```python
from build123d import *

# Parameters (mm, degrees)
SKETCH1_W                                 = 241.3
SKETCH1_H                                 = 177.8
BASE_FLANGE1_DEPTH                        = 3.175
EDGE_FLANGE1_DEPTH                        = 177.8
EDGE_FLANGE1_BEND_DEPTH                   = 177.8
SKETCH13_W                                = 136.525
SKETCH13_H                                = 12.7
BOSS_EXTRUDE1_DEPTH                       = 3.175
SKETCH39_W                                = 136.525
SKETCH39_H                                = 12.7
BOSS_EXTRUDE2_DEPTH                       = 3.175
HOLE_FOR_1_4_SELF_CLINCHING_NUTS_S_SS_C_D = 8.7376
FILLET2_R                                 = 4.7625


# Sheet-metal steps are written as plain solids
with BuildPart() as part:
    # Sketch1 → Base-Flange1 (new body)
    with BuildSketch(Plane(origin=(0, 0, 0), x_dir=(1, 0, 0), z_dir=(0, 1, 0))):
        Rectangle(SKETCH1_W, SKETCH1_H)
    extrude(amount=-BASE_FLANGE1_DEPTH)

    # Edge-Flange1 section (across the edge) → Edge-Flange1 (add)
    with BuildSketch(Plane(origin=(123.825, -3.175, -88.9), x_dir=(-1, 0, 0), z_dir=(0, 0, 1))):
        with BuildLine():
            Line((-3.175, 3.175), (-3.175, 22.225))
            Line((-3.175, 22.225), (0, 22.225))
            Line((0, 22.225), (0, 3.175))
            ThreePointArc((0, 3.175), (0.92993597, 0.92993597), (3.175, 0))
            Line((3.175, 0), (3.175, -3.175))
            ThreePointArc((3.175, -3.175), (-1.315128061, -1.315128061), (-3.175, 3.175))
        make_face()
    extrude(amount=EDGE_FLANGE1_DEPTH)

    # Edge-Flange1 section 2 (across the edge) → Edge-Flange1 bend (add)
    with BuildSketch(Plane(origin=(-123.825, -3.175, 88.9), x_dir=(1, 0, 0), z_dir=(0, 0, -1))):
        with BuildLine():
            Line((-3.175, 3.175), (-3.175, 22.225))
            Line((-3.175, 22.225), (0, 22.225))
            Line((0, 22.225), (0, 3.175))
            ThreePointArc((0, 3.175), (0.92993597, 0.92993597), (3.175, 0))
            Line((3.175, 0), (3.175, -3.175))
            ThreePointArc((3.175, -3.175), (-1.315128061, -1.315128061), (-3.175, 3.175))
        make_face()
    extrude(amount=EDGE_FLANGE1_BEND_DEPTH)

    # Sketch13 → Boss-Extrude1 (add)
    with BuildSketch(Plane(origin=(127, 0, 0), x_dir=(0, 0, -1), z_dir=(1, 0, 0))):
        with Locations((0, -31.75)):
            Rectangle(SKETCH13_W, SKETCH13_H)
    extrude(amount=-BOSS_EXTRUDE1_DEPTH)

    # Sketch39 → Boss-Extrude2 (add)
    with BuildSketch(Plane.ZY.offset(127)):
        with Locations((0, -31.75)):
            Rectangle(SKETCH39_W, SKETCH39_H)
    extrude(amount=-BOSS_EXTRUDE2_DEPTH)

    # Hole for 1/4 Self-clinching Nuts (S,SS,CLS,CLSS)1 (through all)
    with Locations(Plane(origin=(127, 0, 0), x_dir=(0, 0, -1), z_dir=(1, 0, 0))):
        with Locations((-76.2, -15.875), (76.2, -15.875), (58.7375, -28.575), (-49.2125, -28.575)):
            Hole(HOLE_FOR_1_4_SELF_CLINCHING_NUTS_S_SS_C_D / 2)

    # Fillet2
    fillet2_edges = [part.edges().sort_by_distance(p)[0] for p in [
        (125.4125, -25.4, -88.9),
        (125.4125, -25.4, 88.9),
        (-125.4125, -25.4, 88.9),
        (-125.4125, -25.4, -88.9),
        (125.4125, -38.1, -68.2625),
        (125.4125, -25.4, -68.2625),
        (125.4125, -25.4, 68.2625),
        (125.4125, -38.1, 68.2625),
        (-125.4125, -25.4, -68.2625),
        (-125.4125, -38.1, -68.2625),
        (-125.4125, -38.1, 68.2625),
        (-125.4125, -25.4, 68.2625),
    ]]
    fillet(fillet2_edges, radius=FILLET2_R)


solid = part.part
```
Model file for the job. Use its own axes, mm. A direction names the side the tool comes from. Give positions to 0.01 mm unless a question says otherwise; leave off trailing zeros. Order: outer loops, then holes, each group sorted by start corner. A loop starts at its lowest first (then second) coordinate and runs counter-clockwise, first axis right, second up.
1) Saw through at C-C, the plane x = 51.5. Write the cut outline in (y, z) (3 decimals), then the cut area to 3 significant figures.
2) Saw through at A-A, the plane z = 76.2. Write the cut outline in (x, y) (3 decimals), then the cut area to 3 significant figures.
3) Pin check, flat tips, straight feed: pin 1 (2.5 mm diameter, centred on x = -124.5, y = -32, fed in from -Z); pin 2 (5 mm diameter, centred on y = -15.875, z = -76.2, fed in from +X); pin 3 (1.6 mm diameter, centred on x = -126, z = 78.5, fed in from -Y); pin 4 (3.5 mm diameter, centred on x = -125, y = -31.5, fed in from +Z). Stop position of each tip, or through.
4) Mould opens along Z. For faces 1 (the cylindrical face through (-125.435, -24.243, -59.306)), 2 (the cylindrical face through (125.39, -36.74, 66.83)), 3 (the cylindrical face through (125.09, -1.81, -1.24)), 4 (the flat face through (1, -2, -88.9)) say: +Z half, -Z half, draft (parallel to the pull), parting line (faces both ways), or undercut.
5) Saw through at B-B, the plane z = -15. Write the cut outline in (x, y) (3 decimals), then the cut area to 3 significant figures.
6) 3-axis set-ups, long thin cutter, end or side, ignore diameter. For faces 5 (the cylindrical face through (125.39, -18.53, -79.67)), 6 (the flat face through (-2, -3.175, -1)): which of +Z, -Z, +X, -X, +Y, -Y reach the whole face in a straight line?
7) Wall check: probe 1 along X at (y, z) = (-28, -30) (3 decimals); probe 2 along Y at (x, z) = (-89, 5) (3 decimals); probe 3 along X at (y, z) = (-4.5, 11). Give the ranges that are in metal, low to high.
Computed:
1. outline: (-3.175, -88.9) - (0, -88.9) - (0, 88.9) - (-3.175, 88.9) - close
1. area: 565 mm2
2. outline: (-127, -25.4) - (-123.825, -25.4) - (-123.825, -20.244) - (-127, -20.244) - close; (-127, -11.506) - (-123.825, -11.506) - (-123.825, -6.35) arc R3.175 cw to (-120.65, -3.175) - (120.65, -3.175) arc R3.175 cw to (123.825, -6.35) - (123.825, -11.506) - (127, -11.506) - (127, -6.35) arc R6.35 ccw to (120.65, 0) - (-120.65, 0) arc R6.35 ccw to (-127, -6.35) - close; (123.825, -25.4) - (127, -25.4) - (127, -20.244) - (123.825, -20.244) - close
2. area: 879 mm2
3. pin 1: stops at z = -68.26
3. pin 2: passes through
3. pin 3: stops at y = -25.4
3. pin 4: stops at z = 68.28
4. face 1: undercut
4. face 2: +Z half
4. face 3: draft
4. face 4: -Z half
5. outline: (-127, -38.1) - (-123.825, -38.1) - (-123.825, -6.35) arc R3.175 cw to (-120.65, -3.175) - (120.65, -3.175) arc R3.175 cw to (123.825, -6.35) - (123.825, -38.1) - (127, -38.1) - (127, -6.35) arc R6.35 ccw to (120.65, 0) - (-120.65, 0) arc R6.35 ccw to (-127, -6.35) - close
5. area: 1,020 mm2
6. face 5: +X, -X
6. face 6: +Z, -Z, -Y
7. probe 1: x = -127 to -123.825, 123.825 to 127
7. probe 2: y = -3.175 to 0
7. probe 3: x = -126.72 to -123.23, 123.23 to 126.72
